Geometry: final body of the model. Coordinates: model frame, mm. Face numbers are marked on the shaded views. Give positions to 0.01 mm unless a question says otherwise; leave off trailing zeros. Write each loop counter-clockwise with the first axis right and the second up, starting at its lowest first coordinate (ties: lowest second). Pieces come first, ordered by that corner, then holes. Notation, with made-up numbers: (45, -3.75) -> (58, -3.75) arc R17 ccw to (58, 22.25) -> close; hole circle Ø8 at (38.25, 86.25). An arc over 180 degrees is marked (long way). Answer as a JSON object with one key per item and string values. Group by question number.
(1) Section query D-D on x = 3.75. Output: boundary loops of the cut face in (y, z), plus the area to 3 significant figures.
(2) Material intervals for probe 1 along X at (y, z) = (2.3, 0); probe 2 along Z at (x, y) = (1, 3.45); probe 3 along X at (y, z) = (1.1, -1.25), sorted ascending.
(3) Contact query for a flat-ended pin moving along its axis: pin 1 Ø3 at (x, z) = (0, 0) entering from -Y. Output: stop coordinate, or through.
(4) Section query A-A on z = 0. Output: boundary loops of the cut face in (x, y).
(5) Section query B-B on x = 0. Output: boundary loops of the cut face in (y, z).
(6) Section query C-C on y = 3.1. Output: boundary loops of the cut face in (x, z).
(7) Draft query along X for the marked faces 1, 2 and 3. Return one class per face: +X half, -X half, draft (parallel to the pull), parting line (faces both ways), or undercut.
from build123d import *

# Parameters (mm, degrees)
SKETCH1_R           = 5
SKETCH1_R_2         = 2
BOSS_EXTRUDE1_DEPTH = 1.3
SKETCH2_R           = 4.456309589
SKETCH2_R_2         = 2
BOSS_EXTRUDE2_DEPTH = 1.4
LPATTERN2_COUNT     = 2
LPATTERN2_PITCH     = 2.7


with BuildPart() as part:
    # Sketch1 → Boss-Extrude1 (new body)
    with BuildSketch(Plane(origin=(0, 0, 0), x_dir=(1, 0, 0), z_dir=(0, 1, 0))):
        with Locations(Location((0, 0, 0), (0, 0, 270))):
            Circle(SKETCH1_R)
        with Locations(Location((0, 0, 0), (0, 0, 270))):
            Circle(SKETCH1_R_2, mode=Mode.SUBTRACT)
    boss_extrude1 = extrude(amount=BOSS_EXTRUDE1_DEPTH)

    # Sketch2 → Boss-Extrude2 (add)
    with BuildSketch(Plane(origin=(0, 1.3, 0), x_dir=(1, 0, 0), z_dir=(0, 1, 0))):
        with Locations(Location((0, 0, 0), (0, 0, 270))):
            Circle(SKETCH2_R)
        with Locations(Location((0, 0, 0), (0, 0, 270))):
            Circle(SKETCH2_R_2, mode=Mode.SUBTRACT)
    extrude(amount=BOSS_EXTRUDE2_DEPTH)

    # LPattern2: Boss-Extrude1 ×2
    with Locations(*[(0, i * LPATTERN2_PITCH, 0) for i in range(1, LPATTERN2_COUNT)]):
        add(boss_extrude1)


solid = part.part
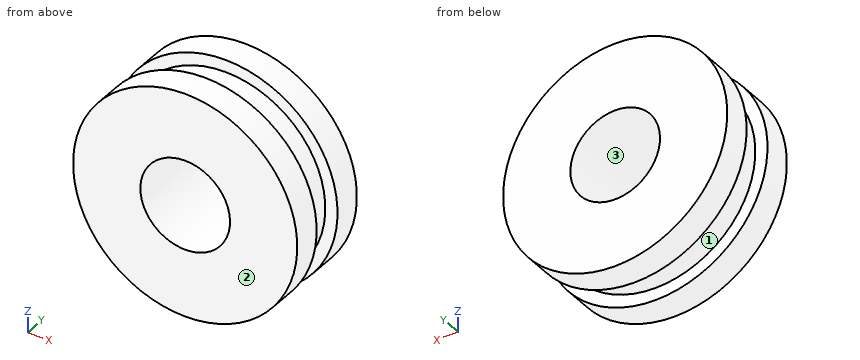
Answer list:
{
 "1": {"outline": "(0, -3.31) -> (1.3, -3.31) -> (1.3, -2.41) -> (2.7, -2.41) -> (2.7, -3.31) -> (4, -3.31) -> (4, 3.31) -> (2.7, 3.31) -> (2.7, 2.41) -> (1.3, 2.41) -> (1.3, 3.31) -> (0, 3.31) -> close", "area": "23.9 mm2"},
 "2": {"probe 1": "-4.46 to -2, 2 to 4.46", "probe 2": "-4.9 to -1.73, 1.73 to 4.9", "probe 3": "-4.84 to -1.56, 1.56 to 4.84"},
 "3": {"pin 1": "through"},
 "4": {"outline": "(-5, 0) -> (-2, 0) -> (-2, 4) -> (-5, 4) -> (-5, 2.7) -> (-4.46, 2.7) -> (-4.46, 1.3) -> (-5, 1.3) -> close; (2, 0) -> (5, 0) -> (5, 1.3) -> (4.46, 1.3) -> (4.46, 2.7) -> (5, 2.7) -> (5, 4) -> (2, 4) -> close"},
 "5": {"outline": "(0, -5) -> (1.3, -5) -> (1.3, -4.46) -> (2.7, -4.46) -> (2.7, -5) -> (4, -5) -> (4, -2) -> (0, -2) -> close; (0, 2) -> (4, 2) -> (4, 5) -> (2.7, 5) -> (2.7, 4.46) -> (1.3, 4.46) -> (1.3, 5) -> (0, 5) -> close"},
 "6": {"outline": "circle Ø10 at (0, 0); hole circle Ø4 at (0, 0)"},
 "7": {"face 1": "parting line", "face 2": "draft", "face 3": "undercut"}
}
